The figure shows three views and two pictorial views of one solid part (mm, origin at its lowest corner). Answer the questions. A direction names the side the tool comes from. Coordinates: 2 decimals unless noted, no trailing zeros. Answer as CSV lines item,"result".
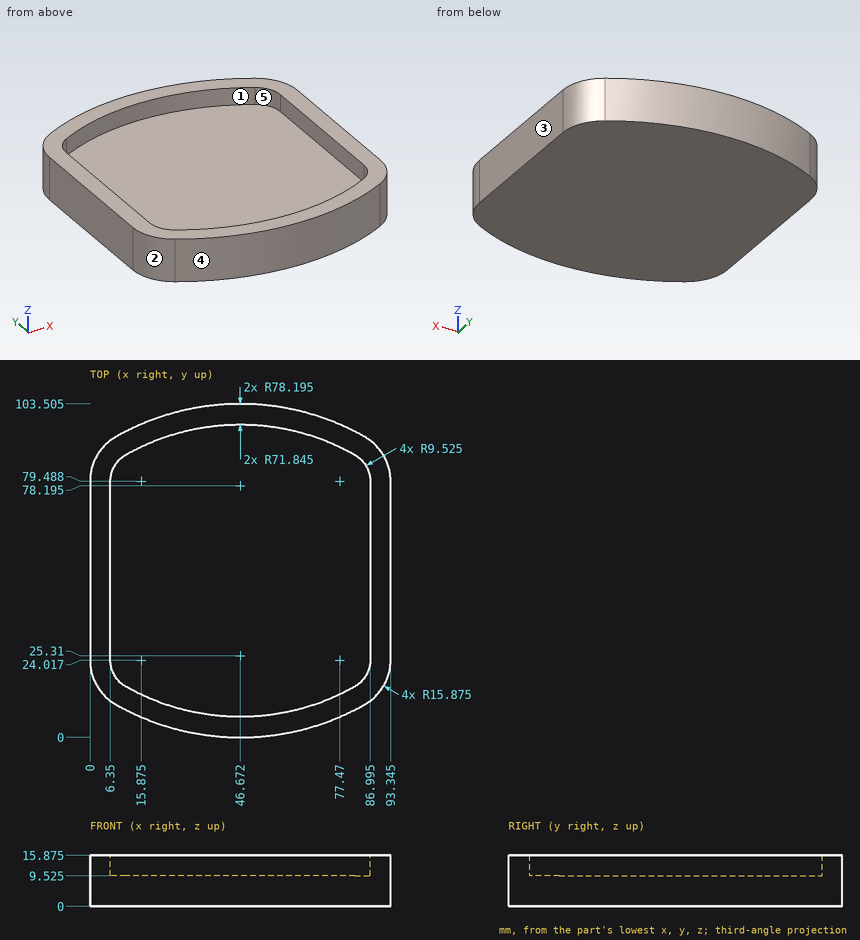
Q1. Straight lines are drawn through the part: line 1 (Y direction, x = 46, z = 14.75); line 2 (Z direction, x = 37.5, y = 36.5) (1 decimal); line 3 (X direction, y = 23.5, z = 9). For each, find the intervals that lie inside material, in ascending order.
Output:
line 1,"0 to 6.35, 97.15 to 103.5"
line 2,"0 to 9.5"
line 3,"0.01 to 93.34"
Q2. Flat-ended cylindrical pins translate along their axes: pin 1 Ø5 at (x, z) = (67, 9.5) entering from -Y; pin 2 Ø5 at (x, z) = (77, 6) entering from -Y; pin 3 Ø1 at (x, y) = (17.5, 33.5) entering from +Z (1 decimal). Find the tip coordinate at first contact, or state that the pin passes through.
Output:
pin 1,"y = 2.06"
pin 2,"y = 5.12"
pin 3,"z = 9.5"
Q3. For the marked faces 1 and 2, determine the directions among +Z, -Z, +X, -X, +Y, -Y from which every point of the face is accessible in a straight line to the end or side of a thin tool.
Output:
face 1,"+Z"
face 2,"+Z, -Z, -X, -Y"
Q4. The mould has two halves that part along Y. Classify the marked faces 3, 4 and 5: pulls with the +Y half, pulls with the -Y half, needs draft (parallel to the pull), parting line crosses it, or undercut.
Output:
face 3,"needs draft"
face 4,"pulls with the -Y half"
face 5,"undercut"
